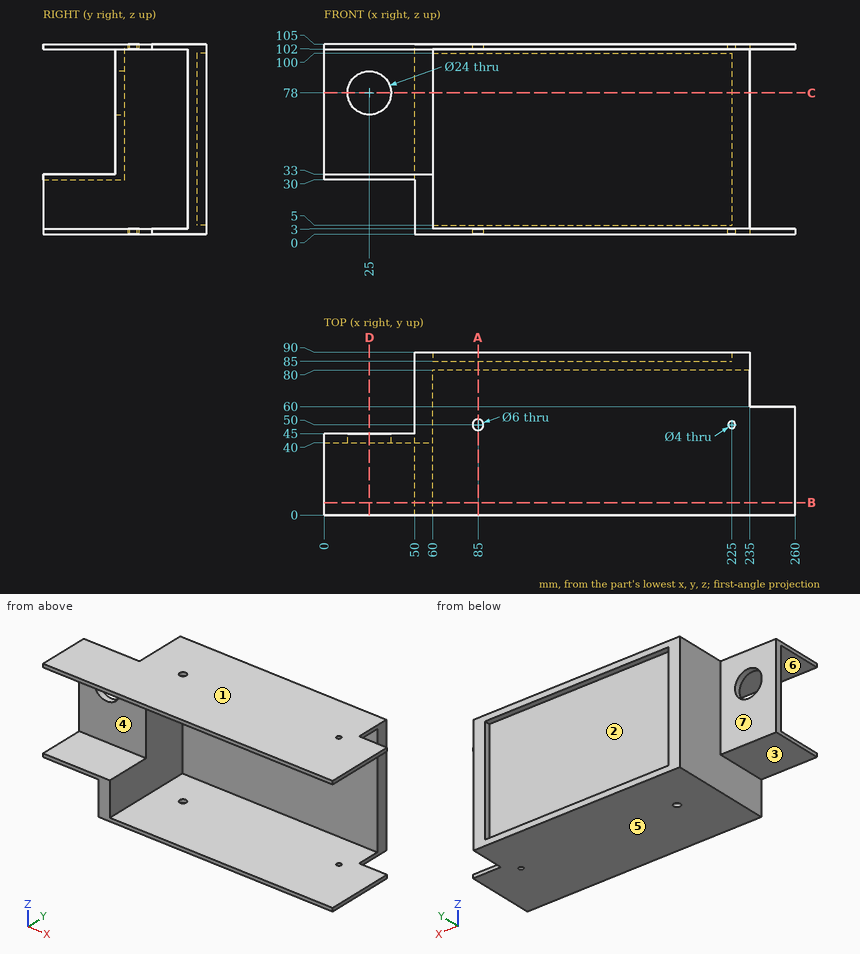
The drawing under review shows one solid part. Ordinate dimensions are in mm from its lowest x, y, z. A direction names the side the tool comes from. Round coordinates to 2 decimals unless told otherwise and drop trailing zeros. Loops run counter-clockwise (first coordinate to the right, second up) from the corner with the lowest first, then second, coordinate; pieces in that order, holes last. Notation, with made-up numbers: (-13, -30) -> (-7, -30) arc R25 cw to (-7, -8) -> close; hole circle Ø3 at (16.25, 20). An arc over 180 degrees is marked (long way). Answer in a Markdown table with one row per item.
1) Consider section A-A, the plane x = 85. Write out the cut boundary in (y, z), plus the area to 3 significant figures.
Taken from the geometry:
| item | result |
|---|---|
| outline | (0, 0) -> (47, 0) -> (47, 3) -> (0, 3) -> close; (0, 102) -> (47, 102) -> (47, 105) -> (0, 105) -> close; (53, 0) -> (90, 0) -> (90, 5) -> (85, 5) -> (85, 100) -> (90, 100) -> (90, 105) -> (53, 105) -> (53, 102) -> (80, 102) -> (80, 3) -> (53, 3) -> close |
| area | 1,020 mm² |
2) Wall thickness on line 1 along Z through (x, y) = (65.5, 33.5); line 2 along Y through (x, z) = (85, 103.05); line 3 along Z through (x, y) = (12.5, 36): over which ranges is each line inside the solid? List them lowest first.
Taken from the geometry:
| item | result |
|---|---|
| line 1 | z = 0 to 3, 102 to 105 |
| line 2 | y = 0 to 47, 53 to 90 |
| line 3 | z = 30 to 33, 102 to 105 |
3) For pin 1 Ø2.5 at (y, z) = (88.5, 29) entering from +X; pin 2 Ø8 at (x, z) = (153, 31) entering from -Y; pin 3 Ø2 at (y, z) = (63.5, 14.5) entering from -X, all flat-tipped, find the tip position at first contact; note any pin that passes through.
Taken from the geometry:
| item | result |
|---|---|
| pin 1 | stops at x = 235 |
| pin 2 | stops at y = 80 |
| pin 3 | stops at x = 50 |
4) Draft analysis for pull direction Z (two halves, no side actions). For the marked faces 1, 2 and 3, state which applies: pulls with the +Z half, pulls with the -Z half, needs draft (parallel to the pull), parting line crosses it, or undercut.
Taken from the geometry:
| item | result |
|---|---|
| face 1 | pulls with the +Z half |
| face 2 | undercut |
| face 3 | pulls with the -Z half |
5) Consider section B-B, the plane y = 7. Write out the cut boundary in (x, z), plus the area to 3 significant figures.
Taken from the geometry:
| item | result |
|---|---|
| outline | (0, 30) -> (50, 30) -> (50, 0) -> (260, 0) -> (260, 3) -> (60, 3) -> (60, 33) -> (0, 33) -> close; (0, 102) -> (260, 102) -> (260, 105) -> (0, 105) -> close |
| area | 1,860 mm² |
6) Consider section D-D, the plane x = 25. Write out the cut boundary in (y, z), plus the area to 3 significant figures.
Taken from the geometry:
| item | result |
|---|---|
| outline | (0, 30) -> (45, 30) -> (45, 66) -> (40, 66) -> (40, 33) -> (0, 33) -> close; (0, 102) -> (40, 102) -> (40, 90) -> (45, 90) -> (45, 105) -> (0, 105) -> close |
| area | 495 mm² |
7) Consider section C-C, the plane z = 78. Write out the cut boundary in (x, y), plus the area to 4 significant figures.
Taken from the geometry:
| item | result |
|---|---|
| outline | (0, 40) -> (13, 40) -> (13, 45) -> (0, 45) -> close; (37, 40) -> (60, 40) -> (60, 80) -> (235, 80) -> (235, 90) -> (225, 90) -> (225, 85) -> (60, 85) -> (60, 90) -> (50, 90) -> (50, 45) -> (37, 45) -> close |
| area | 1,555 mm² |
8) Tool access review of the marked faces 4, 5, 6 and 7: name each direction out of +Z, -Z, +X, -X, +Y, -Y from which nothing blocks a thin tool from reaching the whole face with its end or side.
Taken from the geometry:
| item | result |
|---|---|
| face 4 | +X, -X, -Y |
| face 5 | -Z, +X, -X, +Y, -Y |
| face 6 | +X, -Y |
| face 7 | +Z, -Z, -X, +Y |
